Geometry: see drawing. Coordinates: mm, zero at the bounding-box minimum. Round coordinates to 2 decimals unless told otherwise and drop trailing zeros. Loops run counter-clockwise (first coordinate to the right, second up) from the corner with the lowest first, then second, coordinate; pieces in that order, holes last. Notation, with made-up numbers: (65.5, -8) -> (123.5, -8) arc R22 cw to (123.5, 28) -> close; hole circle Ø8 at (52.25, 62.5). An arc over 180 degrees is marked (long way). Write item = value, one per line.
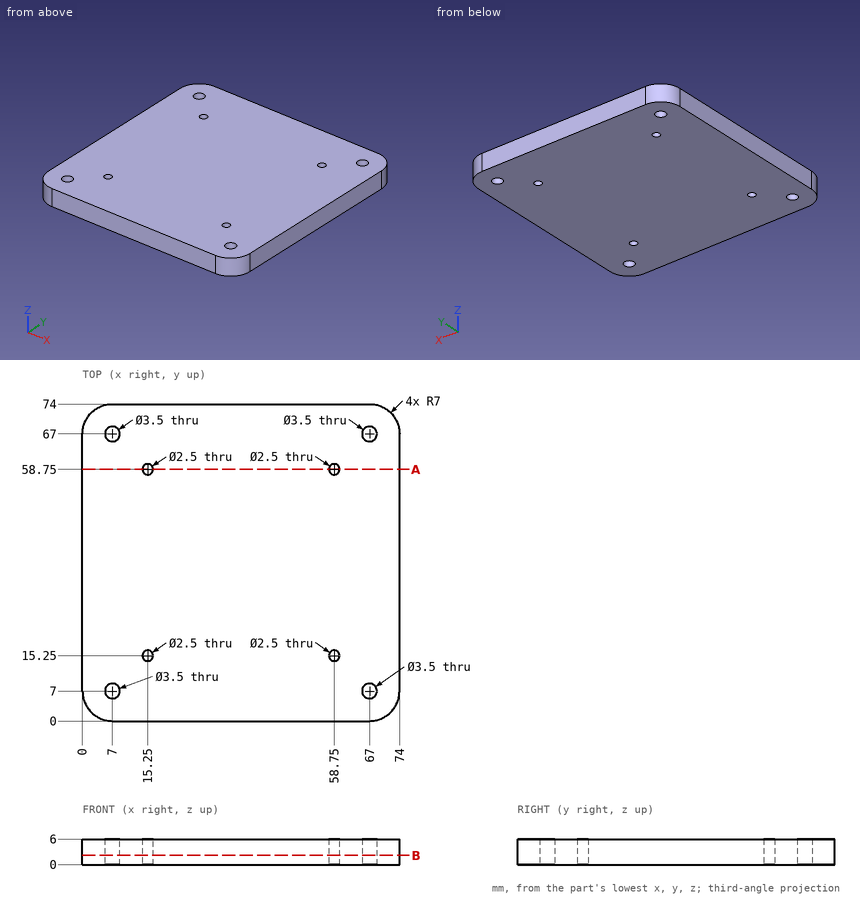
1. Section query B-B (z = 2.2). Give the number of separate pieces and of enclosed holes in the cut face, then the cut area to 3 significant figures.
Evaluation:
separate_pieces = 1
enclosed_holes = 8
area = 5,380 mm²
2. Contact query for a flat-ended pin moving along its axis: pin 1 Ø3 at (x, y) = (67, 7) entering from +Z. Output: stop coordinate, or through.
Evaluation:
pin_1 = through
3. Line query: probe 1 along Y at (x, z) = (7, 2); probe 2 along X at (y, z) = (69, 2.8). Output: solid intervals per line, ascending. Write a range as from..to.
Evaluation:
probe_1 = 0..5.25, 8.75..65.25, 68.75..74
probe_2 = 0.29..73.71
4. Section query A-A (y = 58.75). Return the cut outline in (x, z), then the cut area to 3 significant figures.
Evaluation:
outline = (0, 0) -> (14, 0) -> (14, 6) -> (0, 6) -> close; (16.5, 0) -> (57.5, 0) -> (57.5, 6) -> (16.5, 6) -> close; (60, 0) -> (74, 0) -> (74, 6) -> (60, 6) -> close
area = 414 mm²
